The model under review builds one solid part; all positions refer to its coordinate system, in mm. Coordinates: 2 decimals unless noted, no trailing zeros. Loops run counter-clockwise (first coordinate to the right, second up) from the corner with the lowest first, then second, coordinate; pieces in that order, holes last. Notation, with made-up numbers: M 60.5,89 L 93.5,89 A16 ccw 93.5,106 Z; hole C 35.5,-17.5 d2. An arc over 180 degrees is marked long. Use CSV: the item, a comma, the result in double quotes. Start each with the question number.
from build123d import *

# Parameters (mm, degrees)
F0_W     = 60
F0_H     = 60
F0_R     = 1.75
F0_W_2   = 35
F0_H_2   = 35
F1_DEPTH = 3


with BuildPart() as f1:
    # F0 (on Front) → F1 (new body)
    with BuildSketch(Plane.XZ):
        Rectangle(F0_W, F0_H)
        with Locations((-25, -25)):
            Circle(F0_R, mode=Mode.SUBTRACT)
        with Locations((25, -25)):
            Circle(F0_R, mode=Mode.SUBTRACT)
        with Locations((-25, 25)):
            Circle(F0_R, mode=Mode.SUBTRACT)
        Rectangle(F0_W_2, F0_H_2, mode=Mode.SUBTRACT)
        with Locations((25, 25)):
            Circle(F0_R, mode=Mode.SUBTRACT)
    extrude(amount=F1_DEPTH)


solid = f1.part
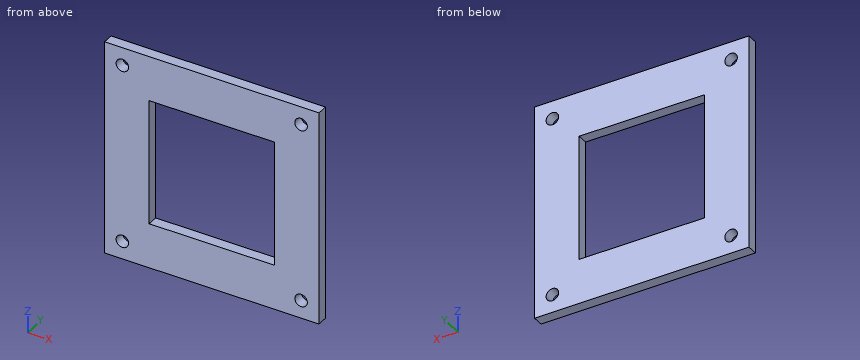
1. Insertion check: pin 1 Ø3 at (x, z) = (25, 25) entering from -Y. The pin has a flat end and moves straight along its axis. Give the tip position at first contact, or say it passes through.
2. To check wall thickness, follow line 1 along Z through (x, y) = (-25, -1.45); line 2 along X through (y, z) = (-0.5, 3). State the ranges of each line that lie inside material, in increasing order.
3. Add section B-B (x = 25). Write out the cut boundary in (y, z).
4. Add section D-D (y = -1.7). Write out the cut boundary in (x, z), plus the area to 3 significant figures.
5. Add section A-A (z = 14.5). Write out the cut boundary in (x, y), plus the area to 3 significant figures.
6. Add section C-C (x = -10). Write out the cut boundary in (y, z), plus the area to 3 significant figures.
Solved:
1,pin 1,"passes through"
2,line 1,"z = -30 to -26.75, -23.25 to 23.25, 26.75 to 30"
2,line 2,"x = -30 to -17.5, 17.5 to 30"
3,outline,"M -3,-30 L 0,-30 L 0,-26.75 L -3,-26.75 Z; M -3,-23.25 L 0,-23.25 L 0,23.25 L -3,23.25 Z; M -3,26.75 L 0,26.75 L 0,30 L -3,30 Z"
4,outline,"M -30,-30 L 30,-30 L 30,30 L -30,30 Z; hole C -25,-25 d3.5; hole C -25,25 d3.5; hole M -17.5,-17.5 L 17.5,-17.5 L 17.5,17.5 L -17.5,17.5 Z; hole C 25,-25 d3.5; hole C 25,25 d3.5"
4,area,"2,340 mm^2"
5,outline,"M -30,-3 L -17.5,-3 L -17.5,0 L -30,0 Z; M 17.5,-3 L 30,-3 L 30,0 L 17.5,0 Z"
5,area,"75.0 mm^2"
6,outline,"M -3,-30 L 0,-30 L 0,-17.5 L -3,-17.5 Z; M -3,17.5 L 0,17.5 L 0,30 L -3,30 Z"
6,area,"75.0 mm^2"
